from build123d import *

# Parameters (mm, degrees)
SKETCH_1_W          = 75
SKETCH_1_H          = 375
EXTRUDE_1_DEPTH     = 25
SKETCH_2_R          = 10.5
CUT_EXTRUDE_1_DEPTH = 26


with BuildPart() as part:
    # Эскиз1 → Бобышка-Вытянуть1 (new body)
    with BuildSketch(Plane.XY):
        with Locations((37.5, 187.5)):
            Rectangle(SKETCH_1_W, SKETCH_1_H)
    extrude(amount=EXTRUDE_1_DEPTH)

    # Эскиз2 → Вырез-Вытянуть1 (cut, through all)
    with BuildSketch(Plane.XY.offset(25)):
        with Locations((37.5, 250)):
            Circle(SKETCH_2_R)
        with Locations((37.5, 300)):
            Circle(SKETCH_2_R)
        with Locations((37.5, 350)):
            Circle(SKETCH_2_R)
        with Locations((37.5, 25)):
            Circle(SKETCH_2_R)
        with BuildLine():
            Line((27, 75), (27, 200))
            ThreePointArc((27, 200), (37.5, 210.5), (48, 200))
            Line((48, 200), (48, 75))
            ThreePointArc((48, 75), (37.5, 64.5), (27, 75))
        make_face()
    extrude(amount=-CUT_EXTRUDE_1_DEPTH, mode=Mode.SUBTRACT)


solid = part.part
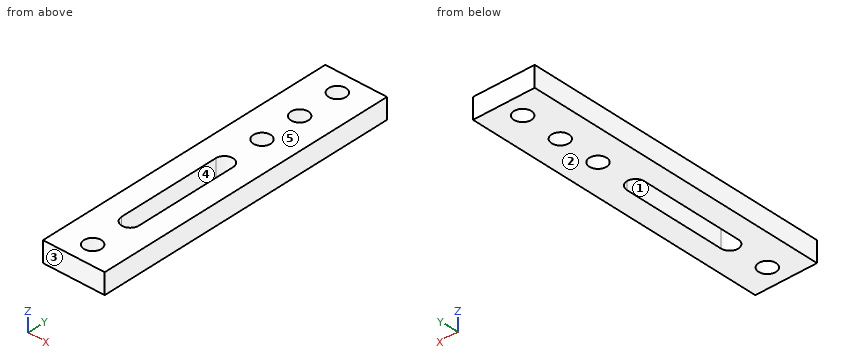
The model under review builds one solid part; all positions refer to its coordinate system, in mm. Face numbers are marked on the shaded views. A direction names the side the tool comes from. Round coordinates to 2 decimals unless told otherwise and drop trailing zeros. Write each loop counter-clockwise with the first axis right and the second up, starting at its lowest first coordinate (ties: lowest second). Pieces come first, ordered by that corner, then holes. Notation, with made-up numbers: M 29,-14.75 L 81,-14.75 A17 ccw 81,2.25 Z; hole C 73.25,25.25 d4. An arc over 180 degrees is marked long. Answer as CSV lines item,"result". Start each with the question number.
Q1. The part is to be moulded in two halves that separate along Y. For the marked faces 1, 2 and 3, say which applies: +Y half, -Y half, draft (parallel to the pull), parting line (faces both ways), or undercut.
Q2. Consider section A-A, the plane y = 350. Give the boundary of the cut face in (x, z).
Q3. Consider section B-B, the plane x = 37.5. Give the boundary of the cut face in (y, z), then the cut area to 4 significant figures.
Q4. Consider section C-C, the plane z = 9.75. Give the boundary of the cut face in (x, y), then the cut area to 3 significant figures.
Q5. Wall thickness on line 1 along Y through (x, z) = (37.5, 13.5); line 2 along X through (y, z) = (150, 21.25); line 3 along Y through (x, z) = (45, 18): over which ranges is each line inside the solid? List them lowest first.
Q6. Clearance check with a flat-ended pin moving along its axis: P1, Ø5, axis at x = 8.5, y = 109.5, coming from the -Z side. State where the tip first meets the part, or that it passes through.
Q7. Tool access review of the marked faces 4 and 5: name each direction out of +Z, -Z, +X, -X, +Y, -Y from which nothing blocks a thin tool from reaching the whole face with its end or side.
Result set:
1,face 1,"undercut"
1,face 2,"draft"
1,face 3,"-Y half"
2,outline,"M 0,0 L 27,0 L 27,25 L 0,25 Z; M 48,0 L 75,0 L 75,25 L 48,25 Z"
3,outline,"M 0,0 L 14.5,0 L 14.5,25 L 0,25 Z; M 35.5,0 L 64.5,0 L 64.5,25 L 35.5,25 Z; M 210.5,0 L 239.5,0 L 239.5,25 L 210.5,25 Z; M 260.5,0 L 289.5,0 L 289.5,25 L 260.5,25 Z; M 310.5,0 L 339.5,0 L 339.5,25 L 310.5,25 Z; M 360.5,0 L 375,0 L 375,25 L 360.5,25 Z"
3,area,"3,625 mm²"
4,outline,"M 0,0 L 75,0 L 75,375 L 0,375 Z; hole C 37.5,25 d21; hole M 27,75 A10.5 ccw 48,75 L 48,200 A10.5 ccw 27,200 Z; hole C 37.5,250 d21; hole C 37.5,300 d21; hole C 37.5,350 d21"
4,area,"23,800 mm²"
5,line 1,"y = 0 to 14.5, 35.5 to 64.5, 210.5 to 239.5, 260.5 to 289.5, 310.5 to 339.5, 360.5 to 375"
5,line 2,"x = 0 to 27, 48 to 75"
5,line 3,"y = 0 to 17.65, 32.35 to 67.65, 207.35 to 242.65, 257.35 to 292.65, 307.35 to 342.65, 357.35 to 375"
6,P1,"stops at z = 0"
7,face 4,"+Z, -Z"
7,face 5,"+Z, +X, -X, +Y, -Y"
